Verification items for this drawing (mm, ordinates from the low corner). A direction names the side the tool comes from. Round coordinates to 2 decimals unless told otherwise and drop trailing zeros. Loops run counter-clockwise (first coordinate to the right, second up) from the corner with the lowest first, then second, coordinate; pieces in that order, holes last. Notation, with made-up numbers: M -6.75,31.25 L 25.25,31.25 A17 cw 25.25,54.25 Z; hole C 11.25,-20.5 d8. An arc over 180 degrees is marked long. Use one line per item in the form item = value. Start each with the question number.
1. Material ranges on line 1 (X direction, y = 7.5, z = 11.25); line 2 (Y direction, x = 8.5, z = 2); line 3 (X direction, y = 2.6, z = 7.5), recorded low to high.
2. Cross-section at A-A (z = 7.5). Record the boundary of the cut face in (x, y).
3. Cross-section at C-C (x = 8.5). Record the boundary of the cut face in (y, z), then the cut area to 3 significant figures.
4. Draft check along Y on the marked faces 4, 5, 6 and 7. Enter one of: pulls with the +Y half, pulls with the -Y half, needs draft (parallel to the pull), parting line crosses it, or undercut.
5. Cross-section at D-D (z = 10.25). Record the boundary of the cut face in (x, y), then the cut area to 3 significant figures.
6. Cross-section at B-B (y = 4.75). Record the boundary of the cut face in (x, z), then the cut area to 3 significant figures.
7. Set-up check for the marked faces 1, 2 and 3: record each of +Z, -Z, +X, -X, +Y, -Y from which the full face is reachable in a straight line by a thin tool's end or side.
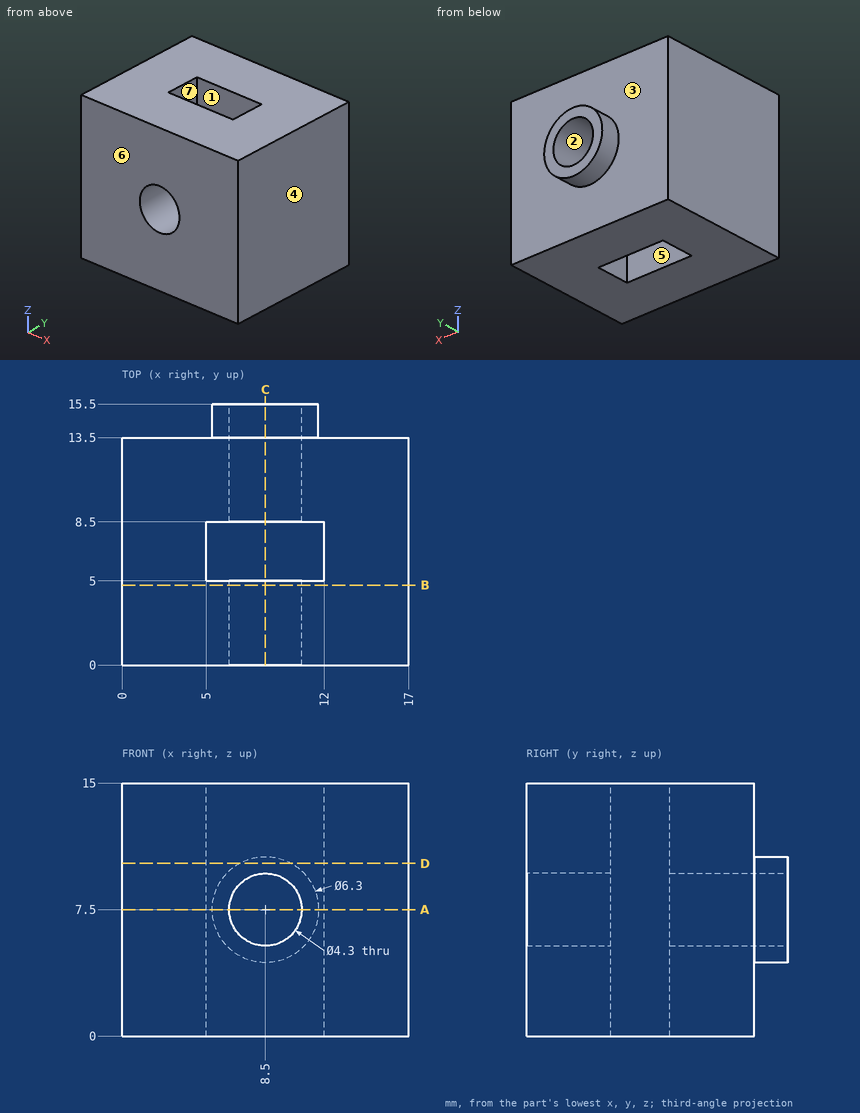
Reported:
q1.line_1 = 0 to 5, 12 to 17
q1.line_2 = 0 to 5, 8.5 to 13.5
q1.line_3 = 0 to 6.35, 10.65 to 17
q2.outline = M 0,0 L 6.35,0 L 6.35,5 L 5,5 L 5,8.5 L 6.35,8.5 L 6.35,15.5 L 5.35,15.5 L 5.35,13.5 L 0,13.5 Z; M 10.65,0 L 17,0 L 17,13.5 L 11.65,13.5 L 11.65,15.5 L 10.65,15.5 L 10.65,8.5 L 12,8.5 L 12,5 L 10.65,5 Z
q3.outline = M 0,0 L 5,0 L 5,5.35 L 0,5.35 Z; M 0,9.65 L 5,9.65 L 5,15 L 0,15 Z; M 8.5,0 L 13.5,0 L 13.5,4.35 L 15.5,4.35 L 15.5,5.35 L 8.5,5.35 Z; M 8.5,9.65 L 15.5,9.65 L 15.5,10.65 L 13.5,10.65 L 13.5,15 L 8.5,15 Z
q3.area = 111 mm²
q4.face_4 = needs draft
q4.face_5 = undercut
q4.face_6 = pulls with the -Y half
q4.face_7 = undercut
q5.outline = M 0,0 L 17,0 L 17,13.5 L 10.04,13.5 L 10.04,15.5 L 6.96,15.5 L 6.96,13.5 L 0,13.5 Z; hole M 5,5 L 12,5 L 12,8.5 L 5,8.5 Z
q5.area = 211 mm²
q6.outline = M 0,0 L 17,0 L 17,15 L 0,15 Z; hole C 8.5,7.5 d4.3
q6.area = 240 mm²
q7.face_1 = +Z, -Z
q7.face_2 = +Y, -Y
q7.face_3 = +Y
